Can you work these out from the model? Positions are in its coordinate system, mm. Face numbers are marked on the shaded views. A direction names the side the tool comes from. Give positions to 0.01 mm unless a question says otherwise; leave off trailing zeros. Answer as CSV lines item,"result".
```python
from build123d import *

# Parameters (mm, degrees)
SKIZZE1_W                          = 24
SKIZZE1_H                          = 10
AUFSATZ_LINEAR_AUSTRAGEN1_DEPTH    = 7
F_4_0_4_DURCHMESSER_BOHRUNG1_D     = 4
F_4_0_4_DURCHMESSER_BOHRUNG1_DEPTH = 5
F_4_0_4_DURCHMESSER_BOHRUNG1_TIP   = 1.201721238
VERRUNDUNG1_SIZE                   = 5
VERRUNDUNG1_SIZE_2                 = 3
FASE2_SIZE                         = 1


with BuildPart() as part:
    # Skizze1 → Aufsatz-Linear austragen1 (new, symmetric)
    with BuildSketch(Plane.XY):
        Rectangle(SKIZZE1_W, SKIZZE1_H)
    extrude(amount=AUFSATZ_LINEAR_AUSTRAGEN1_DEPTH, both=True)

    # Ø4.0 (4) Durchmesser Bohrung1
    with Locations(Plane(origin=(0, 0, -7), x_dir=(-1, 0, 0), z_dir=(0, 0, -1))):
        with Locations((-5.5, 0), (5.5, 0)):
            Hole(F_4_0_4_DURCHMESSER_BOHRUNG1_D / 2, depth=F_4_0_4_DURCHMESSER_BOHRUNG1_DEPTH)
            with Locations((0, 0, -(F_4_0_4_DURCHMESSER_BOHRUNG1_DEPTH + F_4_0_4_DURCHMESSER_BOHRUNG1_TIP / 2))):  # 118° drill point
                Cone(0, F_4_0_4_DURCHMESSER_BOHRUNG1_D / 2, F_4_0_4_DURCHMESSER_BOHRUNG1_TIP, mode=Mode.SUBTRACT)

    # Verrundung1
    # an asymmetric fillet: 5, 3 mm, written as the material it takes off along each edge
    with BuildSketch(Plane(origin=(12, -5, -19.5), x_dir=(-1, 0, 0), z_dir=(0, 0, 1)), Plane(origin=(-12, -5, 19.5), x_dir=(1, 0, 0), z_dir=(0, 0, -1))) as verrundung1_piece_1:
        with BuildLine():
            Bezier((VERRUNDUNG1_SIZE, 0), (0, 0), (0, -VERRUNDUNG1_SIZE_2), weights=[1, 0.707106781, 1])
            Line((0, -VERRUNDUNG1_SIZE_2), (0, 0))
            Line((0, 0), (VERRUNDUNG1_SIZE, 0))
        make_face()
    extrude(amount=39, mode=Mode.SUBTRACT)

    # Fase2
    fase2_edges = [part.edges().sort_by_distance(p)[0] for p in [
        (12, 1.5, 7),
        (10.099176713, -4.354195674, 7),
        (0, -5, 7),
        (-10.099176713, -4.354195674, 7),
        (-12, 1.5, 7),
    ]]
    chamfer(fase2_edges, length=FASE2_SIZE)


solid = part.part
```
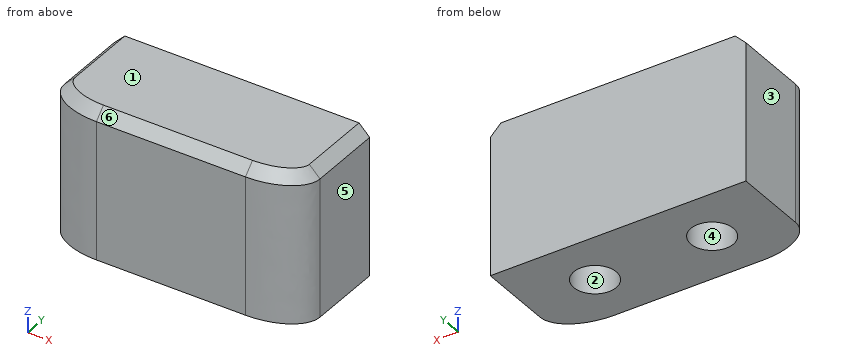
1) I need wall thicknesses on line 1 along X through (y, z) = (0, -3.9); line 2 along Y through (x, z) = (5.5, -4.35); line 3 along Y through (x, z) = (-7.5, -1.25). Which ranges of each line are inside material? Lowest first, please. Write a range as [from, to].
Answer block:
line 1,"[-12, -7.5], [-3.5, 3.5], [7.5, 12]"
line 2,"[-5, -2], [2, 5]"
line 3,"[-4.98, 5]"
2) Which directions (+Z, -Z, +X, -X, +Y, -Y) give clear straight access to the entire face, cutting with the end or side of a thin tool? Please do the marked faces 1 and 2.
Answer block:
face 1,"+Z, +X, -X, +Y, -Y"
face 2,"-Z"
3) If we mould it in two halves opening along X, with no side actions, what happens to the marked faces 3, 4, 5 and 6? For each: +X half, -X half, draft (parallel to the pull), parting line (faces both ways), or undercut.
Answer block:
face 3,"-X half"
face 4,"undercut"
face 5,"+X half"
face 6,"draft"
